Source: CAD feature listing. Evaluate the final solid. Frame: model axes, mm. A direction names the side the tool comes from. Coordinates: 2 decimals unless noted, no trailing zeros. Order: outer loops, then holes, each group sorted by start corner. A loop starts at its lowest first (then second) coordinate and runs counter-clockwise, first axis right, second up.
Autodesk Inventor part; units mm, degrees
ref_plane "YZ Plane" through (0, 0, 0) normal (1, 0, 0) x (0, 1, 0)
ref_plane "XZ Plane" through (0, 0, 0) normal (0, 1, 0) x (-1, 0, 0)
ref_plane "XY Plane" through (0, 0, 0) normal (0, 0, 1) x (1, 0, 0)
sketch "Sketch1" plane through (0, 0, 0) normal (0, 1, 0) x (-1, 0, 0)
  circle A0 centre (0, 0) radius 14
  circle A1 centre (0, 0) radius 13
  circle A2 centre (0, 0) radius 16
  dimension "d0" = 26
  dimension "d1" = 28
  dimension "d2" = 32
extrude "Extrusion1" add sketch "Sketch1" along normal blind 22.5 contours A0 | A2
extrude "Extrusion2" cut sketch "Sketch1" along normal blind 8 contours A0
mirror "Mirror1" about plane through (0, 22.5, 0) normal (0, 1, 0)
equation "\"d0\" = CsapágyHázBelsőÁtmérő"
equation "\"d1\" = CsapágyKülsőÁtmérő"
equation "\"d2\" = CsapágyHázKülsőÁtmérő"
equation "\"d3\" = 0.5 * CsapágyHázHoszza"
equation "\"d5\" = CsapágySzélesége"
equation "\"ZártSzelvényFalVastagság\" = 1.5"
equation "\"ZártSzelvényBelsőÁtmérő\" = 12"
equation "\"ZártSzelvényKülsőÁtmérő\" = 15"
equation "\"CsapágyBelsőÁtmérő\" = 12"
equation "\"CsapágySzélesége\" = 8"
equation "\"CsapágyKülsőÁtmérő\" = 28"
equation "\"CsapágyHázBelsőÁtmérő\" = 26"
equation "\"CsapágyHázHoszza\" = 45"
equation "\"CsapágyHázKülsőÁtmérő\" = 32"
properties part number "CsapágyHáz" material "Acetal Resin, Black"
1. Access query for faces 1 (the face through (10.316, 22.297, 7.91)), 2 (the face through (-12.932, 3.944, 5.362)), 3 (the face through (9.3, 37, -9.3)). Directions: +Z, -Z, +X, -X, +Y, -Y. A direction counts if a zero-diameter tool reaches every point of the face in a straight line with its end or side. Return the directions, or none.
Findings:
face 1: +Y, -Y
face 2: -Y
face 3: +Y
2. Section query B-B on z = 0. Return loops of the section in (x, y).
Findings:
outline: (-16, 0) - (-14, 0) - (-14, 8) - (-13, 8) - (-13, 37) - (-14, 37) - (-14, 45) - (-16, 45) - close; (13, 8) - (14, 8) - (14, 0) - (16, 0) - (16, 45) - (14, 45) - (14, 37) - (13, 37) - close
3. Draft query along Z for faces 4 (the face through (3.47, 22.18, 15.62)), 5 (the face through (-0.07, 45, -14.15)), 6 (the face through (-9.3, 8, -9.3)). Return one class per face: released by +Z, released by -Z, zero draft, split by the parting line, or undercut.
Findings:
face 4: split by the parting line
face 5: zero draft
face 6: undercut
4. Ray query, line 1 (Z direction, x = 0, y = 4.75); line 2 (Z direction, x = -0.5, y = 36); line 3 (X direction, y = 13.5, z = 8). Return the intervals inside material, ascending.
Findings:
line 1: z = -16 to -14, 14 to 16
line 2: z = -15.99 to -12.99, 12.99 to 15.99
line 3: x = -13.86 to -10.25, 10.25 to 13.86
5. Section query A-A on x = 0. Return loops of the section in (y, z), plus the area to 3 significant figures.
Findings:
outline: (0, -16) - (45, -16) - (45, -14) - (37, -14) - (37, -13) - (8, -13) - (8, -14) - (0, -14) - close; (0, 14) - (8, 14) - (8, 13) - (37, 13) - (37, 14) - (45, 14) - (45, 16) - (0, 16) - close
area: 238 mm2
6. Pin query (flat end, axial travel): P1, Ø1, axis at x = -5.5, y = 12, coming from the +Z side; P2, Ø1.5, axis at x = 12.5, y = 38, coming from the -Z side; P3, Ø8, axis at y = 18, z = -12.5, coming from the +X side; P4, Ø2, axis at x = -10.5, z = -2, coming from the -Y side. Return the tip coordinate at first contact, or that it passes through.
Findings:
P1: stops at z = 15.2
P2: stops at z = -10.86
P3: stops at x = 13.56
P4: passes through
7. Section query C-C on y = 10. Return loops of the section in (x, z), plus the area to 3 significant figures.
Findings:
outline: circle Ø32 at (0, 0); hole circle Ø26 at (0, 0)
area: 273 mm2
